from build123d import *

# Parameters (mm, degrees)
FILLET1_R      = 0.79375
CHAMFER1_SIZE  = 0.79375
CHAMFER1_SIZE2 = 1.374815329


with BuildPart() as part:
    # Sketch1 → Revolve1 (revolve)
    with BuildSketch(Plane.XY):
        Polygon((0, 0), (-9.398, 0), (-9.398, 1.5875), (-7.112, 4.445), (-7.112, 7.62), (-9.398, 7.62), (-9.398, 12.7), (0, 12.7), align=None)
    revolve(axis=Axis((0, 0, 0), (0, 1, 0)))

    # Fillet1
    fillet1_edges = [part.edges().sort_by_distance(p)[0] for p in [
        (9.398, 0, 0),
    ]]
    fillet(fillet1_edges, radius=FILLET1_R)

    # Chamfer1
    chamfer1_edges = [part.edges().sort_by_distance(p)[0] for p in [
        (9.398, 12.7, 0),
    ]]
    chamfer1_side = [part.faces().sort_by_distance(p)[0] for p in [
        (0, 12.7, 0),
    ]]
    chamfer(chamfer1_edges, length=CHAMFER1_SIZE, length2=CHAMFER1_SIZE2, reference=chamfer1_side[0])


solid = part.part
Check sheet for the modelled part. Datum: model origin and axes. Units: mm. A direction names the side the tool comes from. Round coordinates to 2 decimals unless told otherwise and drop trailing zeros. Order: outer loops, then holes, each group sorted by start corner. A loop starts at its lowest first (then second) coordinate and runs counter-clockwise, first axis right, second up.
Q1. Draft check along Y on faces 3 (the face through (1.22, 1.2, 9.32)), 4 (the face through (0, 12.7, 0)), 5 (the face through (-7, 7.62, 2)), 6 (the face through (0, 0, 0)). Enter one of: pulls with the +Y half, pulls with the -Y half, needs draft (parallel to the pull), parting line crosses it, or undercut.
Filled sheet:
face 3: needs draft
face 4: pulls with the +Y half
face 5: undercut
face 6: pulls with the -Y half
Q2. Cross-section at D-D, the plane y = 8.5. Enter the section's corners in (x, z).
Filled sheet:
outline: circle Ø18.8 at (0, 0)
Q3. Cross-section at C-C, the plane y = 6.25. Enter the section's corners in (x, z).
Filled sheet:
outline: circle Ø14.22 at (0, 0)
Q4. Cross-section at B-B, the plane x = 0. Enter the section's corners in (y, z) (1 decimal).
Filled sheet:
outline: (0, -8.6) arc R0.8 ccw to (0.8, -9.4) - (1.6, -9.4) - (4.4, -7.1) - (7.6, -7.1) - (7.6, -9.4) - (11.3, -9.4) - (12.7, -8.6) - (12.7, 8.6) - (11.3, 9.4) - (7.6, 9.4) - (7.6, 7.1) - (4.4, 7.1) - (1.6, 9.4) - (0.8, 9.4) arc R0.8 ccw to (0, 8.6) - close
Q5. Depth check by flat-ended pin: P1, Ø3, axis at x = 3, y = 10.5, coming from the -Z side; P2, Ø5, axis at x = 7, y = 9, coming from the +Z side; P3, Ø1, axis at y = 1.5, z = -3.5, coming from the +X side. Enter the tip coordinate at first touch or a pass-through.
Filled sheet:
P1: stops at z = -9.28
P2: stops at z = 8.25
P3: stops at x = 8.91
Q6. Cross-section at A-A, the plane z = 0. Enter the section's corners in (x, y) (1 decimal), plus the area to 3 significant figures.
Filled sheet:
outline: (-9.4, 0.8) arc R0.8 ccw to (-8.6, 0) - (8.6, 0) arc R0.8 ccw to (9.4, 0.8) - (9.4, 1.6) - (7.1, 4.4) - (7.1, 7.6) - (9.4, 7.6) - (9.4, 11.3) - (8.6, 12.7) - (-8.6, 12.7) - (-9.4, 11.3) - (-9.4, 7.6) - (-7.1, 7.6) - (-7.1, 4.4) - (-9.4, 1.6) - close
area: 216 mm2
Q7. Scan lines: L1, parallel to X at y = 5, z = 0.25; L2, parallel to Y at x = 7, z = -2.5; L3, parallel to Y at x = -1, z = -7.25. Record each from-to range of solid material in increasing order.
Filled sheet:
L1: x = -7.11 to 7.11
L2: y = 0 to 4.04, 7.62 to 12.7
L3: y = 0 to 4.19, 7.62 to 12.7
Q8. Set-up check for faces 1 (the face through (1.22, 9.5, 9.32)), 2 (the face through (1.542, 6.055, -6.943)): record each of +Z, -Z, +X, -X, +Y, -Y from which the full face is reachable in a straight line by a thin tool's end or side.
Filled sheet:
face 1: +Y, -Y
face 2: none
